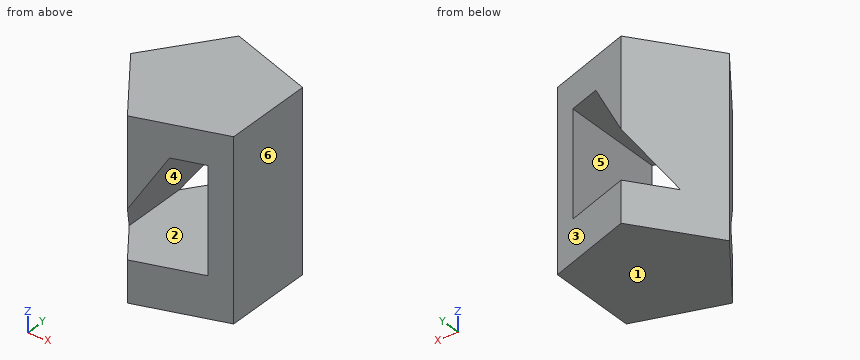
from build123d import *

# Parameters (mm, degrees)
F1_DEPTH = 38.1
F3_DEPTH = 27.686


with BuildPart() as f1:
    # F0 (on Top) → F1 (new body)
    with BuildSketch(Plane.XY):
        Polygon((13.172377, -9.570292), (13.172377, 9.570292), (-5.0314, 15.485058), (-16.281953, 0), (-5.0314, -15.485058), align=None)
    extrude(amount=F1_DEPTH)

    # F2 (on Front) → F3 (cut, symmetric)
    with BuildSketch(Plane.XZ):
        Polygon((8.781587, 31.223414), (2.195396, 31.223414), (-11.220914, 8.781586), (8.781587, 8.781586), align=None)
    extrude(amount=F3_DEPTH, both=True, mode=Mode.SUBTRACT)


solid = f1.part
CAD build for the part. Positions are in the model's coordinates, mm. Face numbers are marked on the shaded views. A direction names the side the tool comes from. Give positions to 0.01 mm unless a question says otherwise; leave off trailing zeros. Write each loop counter-clockwise with the first axis right and the second up, starting at its lowest first coordinate (ties: lowest second). Pieces come first, ordered by that corner, then holes. Notation, with made-up numbers: M 80,4.5 L 114,4.5 A19 cw 114,22.5 Z; hole C -29,44 d4. An arc over 180 degrees is marked long. Put each result on its own line as item: value. Start each with the question number.
(1) Band-saw the part on A-A, the plane z = 15.5. Write the cut outline in (x, y).
(2) Probe L1, parallel to Z at x = 1, y = -7; L2, parallel to Z at x = 6.5, y = 11.5; L3, parallel to X at y = 8, z = 13.5. List the from-to ranges inside material, lowest first.
(3) Band-saw the part on D-D, the plane y = 12. Write the cut outline in (x, z), and give its area (3 significant figures).
(4) Band-saw the part on C-C, the plane y = 4. Write the cut outline in (x, z), and give its area (3 significant figures).
(5) Flat gauge pins, fed straight in: pin 1 Ø10 at (x, z) = (1, 5) entering from +Y; pin 2 Ø12 at (x, z) = (-12.5, 29) entering from -Y. Where does each tip first touch, or does it go through?
(6) Which spindle directions (+Z, -Z, +X, -X, +Y, -Y) get a long thin tool onto all of the face, cutting with end or side? Do the marked faces 5 and 6. Say none if no direction does.
(7) Mould opens along Z. For the marked faces 1, 2, 3 and 4 say: +Z half, -Z half, draft (parallel to the pull), parting line (faces both ways), or undercut.
(8) Band-saw the part on B-B, the plane x = -8.75. Write the cut outline in (y, z).
Response values:
1. outline: M -16.28,0 L -7.2,-12.49 L -7.2,12.49 Z; M 8.78,-11 L 13.17,-9.57 L 13.17,9.57 L 8.78,11 Z
2. L1: z = 0 to 8.78, 29.22 to 38.1
2. L2: z = 0 to 8.78, 31.22 to 38.1
2. L3: x = -10.47 to -8.4, 8.78 to 13.17
3. outline: M -7.56,0 L 5.69,0 L 5.69,8.78 L -7.56,8.78 Z; M -7.56,14.9 L 2.2,31.22 L 5.69,31.22 L 5.69,38.1 L -7.56,38.1 Z
3. area: 287 mm2
4. outline: M -13.38,0 L 13.17,0 L 13.17,38.1 L -13.38,38.1 Z; hole M -11.22,8.78 L 8.78,8.78 L 8.78,31.22 L 2.2,31.22 Z
4. area: 713 mm2
5. pin 1: stops at y = 15.15
5. pin 2: stops at y = -13.46
6. face 5: +Y, -Y
6. face 6: +Z, -Z, +X, +Y, -Y
7. face 1: -Z half
7. face 2: undercut
7. face 3: draft
7. face 4: undercut
8. outline: M -10.37,0 L 10.37,0 L 10.37,8.78 L -10.37,8.78 Z; M -10.37,12.91 L 10.37,12.91 L 10.37,38.1 L -10.37,38.1 Z
